Could you check a few things on this drawing? It's one solid part, dimensions in mm from its lowest x, y, z. A direction names the side the tool comes from. Give positions to 0.01 mm unless a question says otherwise; leave off trailing zeros. Loops run counter-clockwise (first coordinate to the right, second up) from the corner with the lowest first, then second, coordinate; pieces in that order, holes last. Notation, with made-up numbers: (10, -8.5) -> (43, -8.5) arc R15 ccw to (43, 14.5) -> close; hole circle Ø11 at (83, -1.5). An arc over 180 degrees is marked (long way). Use CSV: the item, a comma, the result in double quotes.
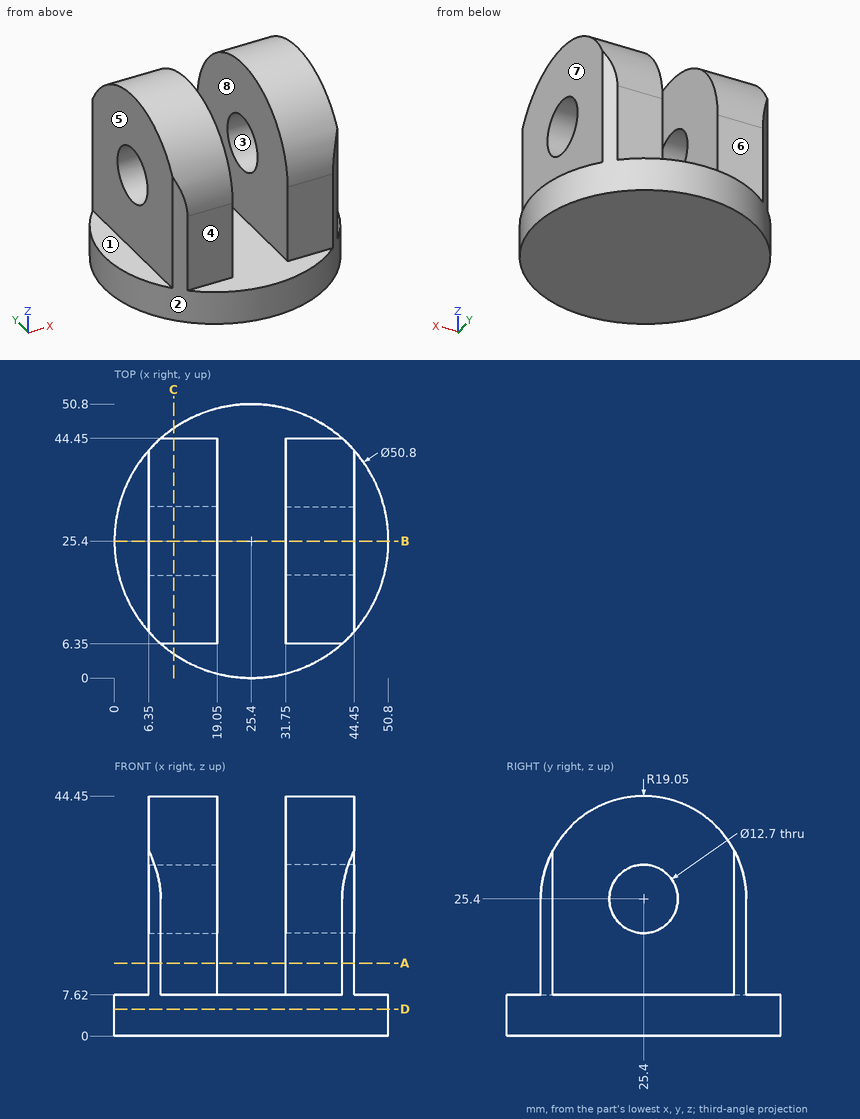
(1) If we section it at A-A, the plane z = 13.5: Write out the boundary of the cut face in (x, y), then the cut area to 3 significant figures.
Answer sheet:
outline,"(6.35, 8.6) arc R25.4 ccw to (8.6, 6.35) -> (19.05, 6.35) -> (19.05, 44.45) -> (8.6, 44.45) arc R25.4 ccw to (6.35, 42.2) -> close; (31.75, 6.35) -> (42.2, 6.35) arc R25.4 ccw to (44.45, 8.6) -> (44.45, 42.2) arc R25.4 ccw to (42.2, 44.45) -> (31.75, 44.45) -> close"
area,"958 mm2"
(2) We'd pull the mould along Y, two halves only. Please class the marked faces 1, 2 and 3: released by +Y, released by -Y, zero draft, split by the parting line, or undercut.
Answer sheet:
face 1,"zero draft"
face 2,"split by the parting line"
face 3,"undercut"
(3) If we section it at B-B, the plane y = 25.4: Write out the boundary of the cut face in (x, z), then the cut area to 4 significant figures.
Answer sheet:
outline,"(0, 0) -> (50.8, 0) -> (50.8, 7.62) -> (44.45, 7.62) -> (44.45, 19.05) -> (31.75, 19.05) -> (31.75, 7.62) -> (19.05, 7.62) -> (19.05, 19.05) -> (6.35, 19.05) -> (6.35, 7.62) -> (0, 7.62) -> close; (6.35, 31.75) -> (19.05, 31.75) -> (19.05, 44.45) -> (6.35, 44.45) -> close; (31.75, 31.75) -> (44.45, 31.75) -> (44.45, 44.45) -> (31.75, 44.45) -> close"
area,"1,000 mm2"
(4) Which directions (+Z, -Z, +X, -X, +Y, -Y) give clear straight access to the entire face, cutting with the end or side of a thin tool? Please do the marked faces 4, 5, 6, 7 and 8.
Answer sheet:
face 4,"+Z, +X, -X, -Y"
face 5,"+Z, -X, +Y, -Y"
face 6,"+Z, +X, -X, +Y"
face 7,"+Z, +X, +Y, -Y"
face 8,"+Z, +Y, -Y"
(5) If we section it at C-C, the plane x = 11: Write out the boundary of the cut face in (y, z), then the cut area to 3 significant figures.
Answer sheet:
outline,"(4.48, 0) -> (46.32, 0) -> (46.32, 7.62) -> (44.45, 7.62) -> (44.45, 25.4) arc R19.05 ccw to (6.35, 25.4) -> (6.35, 7.62) -> (4.48, 7.62) -> close; hole circle Ø12.7 at (25.4, 25.4)"
area,"1,440 mm2"
(6) Will these pins go through, and if not, where does the flat tip stop? pin 1 Ø12 at (x, z) = (41.5, 5.5) entering from +Y; pin 2 Ø3 at (x, z) = (35.5, 19) entering from +Y; pin 3 Ø1 at (x, z) = (26.5, 6.5) entering from +Y; pin 4 Ø10 at (y, z) = (25.4, 25.4) entering from +X.
Answer sheet:
pin 1,"stops at y = 48.71"
pin 2,"stops at y = 44.45"
pin 3,"stops at y = 50.79"
pin 4,"passes through"
(7) If we section it at D-D, the plane z = 5: Write out the boundary of the cut face in (x, y), then the cut area to 3 significant figures.
Answer sheet:
outline,"circle Ø50.8 at (25.4, 25.4)"
area,"2,030 mm2"
(8) If I drill on L1, parallel to Z at x = 15, y = 25; L2, parallel to X at y = 32.5, z = 23; L3, parallel to Y at x = 14, z = 25, over which ranges is the centre line in solid material (lowest first)? Write a range as from..to.
Answer sheet:
L1,"z = 0..19.06, 31.74..44.45"
L2,"x = 6.35..19.05, 31.75..44.45"
L3,"y = 6.35..19.06, 31.74..44.45"
